Input: part model. Units: mm. Frame: model coordinates. A direction names the side the tool comes from. Give positions to 0.01 mm unless a question says otherwise; leave off trailing zeros. Write each loop counter-clockwise with the first axis right and the second up, starting at its lowest first coordinate (ties: lowest second). Pieces come first, ordered by that corner, then holes. Notation, with made-up numbers: (-37.5, 75.25) - (-20.5, 75.25) arc R31 cw to (-20.5, 113.25) - close; hole circle Ø4 at (56, 27.25). An arc over 180 degrees is marked (long way). Use a Markdown table: item, result. Add a question column.
1. Section query B-B, the plane z = 4.5. Return loops of the section in (x, y).
2. Set-up query: faces 1 (the cylindrical face through (29.94, -24.34, -225.24)), 2 (the cylindrical face through (4.877, -30.068, -17.07)), 3 (the cylindrical face through (-2.912, 27.277, 22.51)), 4 (the flat face through (8, -26, 58)), 5 (the flat face through (-2, -32.3, -485)). Return all of +Z, -Z, +X, -X, +Y, -Y with unobstructed straight access to the full face (end or side cutting, diameter ignored); none if empty.
3. Mould query, pull axis Z, two halves, no side actions, for faces 6 (the flat face through (-23, 7, -436.519)), 7 (the cylindrical face through (-11.95, -19.52, -232.16)), 8 (the flat face through (-11, -26, -516.519)). Classes: released by +Z, released by -Z, zero draft, split by the parting line, or undercut.
4. Pin query (flat end, axial travel): pin 1 (1.9 mm diameter, centred on y = -30.5, z = -478, fed in from -X); pin 2 (2 mm diameter, centred on y = 27.5, z = -390, fed in from +X); pin 3 (3 mm diameter, centred on y = -30, z = 25.5, fed in from +X). Return the tip coordinate at first contact, or that it passes through.
5. Section query C-C, the plane y = 0. Return loops of the section in (x, z), plus the area to 3 significant figures.
6. Section query D-D, the plane z = -226. Return loops of the section in (x, y), plus the area to 3 significant figures.
7. Section query A-A, the plane x = -1.8. Return loops of the section in (y, z), plus the area to 3 significant figures.
8. Material intervals for probe 1 along Z at (x, y) = (8.5, 28); probe 2 along Y at (x, z) = (-1.8, -489.5); probe 3 along Y at (x, z) = (-1.8, -16.25), sorted ascending.
```python
from build123d import *

# Parameters (mm, degrees)
CUT_EXTRUDE1_DEPTH      = 10
CUT_EXTRUDE1_DEPTH_BACK = 5


with BuildPart() as part:
    # Sketch1 → Revolve1 (revolve)
    with BuildSketch(Plane.XZ, mode=Mode.PRIVATE) as revolve1_sk:
        Polygon((38.2, -516.518644329), (38.2, 57.999999671), (25.5, 57.999999671), (25.5, -12.000000329), (29, -12.000000329), (29, -22.000000329), (20.2, -22.000000329), (20.2, -436.518644329), (29, -436.518644329), (29, -446.518644329), (25.5, -446.518644329), (25.5, -516.518644329), align=None)
    revolve(revolve1_sk.sketch.rotate(Axis((-1.8, 0, 70), (0, 0, -1)), 180), axis=Axis((-1.8, 0, 70), (0, 0, -1)))

    # Sketch3 → Cut-Extrude1 (cut, two sides: drawn at the far end of the back side and taken through both)
    with BuildSketch(Plane(origin=(0, -27.3, 0), x_dir=(1, 0, 0), z_dir=(0, 1, 0)).offset(-CUT_EXTRUDE1_DEPTH_BACK)):
        with BuildLine():
            Line((6.2, 521.518644329), (6.2, 461.518644329))
            ThreePointArc((6.2, 461.518644329), (-1.8, 453.518644329), (-9.8, 461.518644329))
            Line((-9.8, 461.518644329), (-9.8, 521.518644329))
            ThreePointArc((-9.8, 521.518644329), (-1.8, 529.518644329), (6.2, 521.518644329))
        make_face()
        with BuildLine():
            Line((-9.8, -53.000000001), (-9.8, 6.999999999))
            ThreePointArc((-9.8, 6.999999999), (-1.8, 14.999999999), (6.2, 6.999999999))
            Line((6.2, 6.999999999), (6.2, -53.000000001))
            ThreePointArc((6.2, -53.000000001), (-1.8, -61.000000001), (-9.8, -53.000000001))
        make_face()
    extrude(amount=CUT_EXTRUDE1_DEPTH + CUT_EXTRUDE1_DEPTH_BACK, mode=Mode.SUBTRACT)


solid = part.part
```
Result sheet:
| question | item | result |
|---|---|---|
| 1 | outline | circle Ø80 at (-1.8, 0); hole (-9.8, -32.3) - (6.2, -32.3) - (6.2, -26.1) arc R27.3 ccw (long way) to (-9.8, -26.1) - close |
| 2 | face 1 | +Z, -Z |
| 2 | face 2 | none |
| 2 | face 3 | +Z |
| 2 | face 4 | +Z, +X, -X, +Y, -Y |
| 2 | face 5 | -Z |
| 3 | face 6 | undercut |
| 3 | face 7 | zero draft |
| 3 | face 8 | released by -Z |
| 4 | pin 1 | stops at x = -28.76 |
| 4 | pin 2 | stops at x = 28.16 |
| 4 | pin 3 | stops at x = 26.27 |
| 5 | outline | (-41.8, -516.52) - (-29.1, -516.52) - (-29.1, -446.52) - (-32.6, -446.52) - (-32.6, -436.52) - (-23.8, -436.52) - (-23.8, -22) - (-32.6, -22) - (-32.6, -12) - (-29.1, -12) - (-29.1, 58) - (-41.8, 58) - close; (20.2, -436.52) - (29, -436.52) - (29, -446.52) - (25.5, -446.52) - (25.5, -516.52) - (38.2, -516.52) - (38.2, 58) - (25.5, 58) - (25.5, -12) - (29, -12) - (29, -22) - (20.2, -22) - close |
| 5 | area | 18,800 mm² |
| 6 | outline | circle Ø80 at (-1.8, 0); hole circle Ø44 at (-1.8, 0) |
| 6 | area | 3,510 mm² |
| 7 | outline | (-40, -516.52) - (-32.3, -516.52) - (-32.3, -453.52) - (-27.3, -453.52) - (-27.3, -446.52) - (-30.8, -446.52) - (-30.8, -436.52) - (-22, -436.52) - (-22, -22) - (-30.8, -22) - (-30.8, -15) - (-32.3, -15) - (-32.3, 58) - (-40, 58) - close; (22, -436.52) - (30.8, -436.52) - (30.8, -446.52) - (27.3, -446.52) - (27.3, -516.52) - (40, -516.52) - (40, 58) - (27.3, 58) - (27.3, -12) - (30.8, -12) - (30.8, -22) - (22, -22) - close |
| 7 | area | 18,200 mm² |
| 8 | probe 1 | z = -516.52 to -446.52, -436.52 to -22, -12 to 58 |
| 8 | probe 2 | y = -40 to -32.3, 27.3 to 40 |
| 8 | probe 3 | y = -40 to -30.8, 30.8 to 40 |
